```python
from build123d import *

# Parameters (mm, degrees)
ESBO_O1_R                = 2.95
RESSALTO_EXTRUS_O1_DEPTH = 1.4
CORTE_EXTRUS_O1_START    = -1
CORTE_EXTRUS_O1_DEPTH    = 1
ESBO_O3_R                = 2.1
RESSALTO_EXTRUS_O2_DEPTH = 1
FILETE3_R                = 0.2
ESBO_O4_R                = 2
RESSALTO_EXTRUS_O3_DEPTH = 6.5
FILETE4_R                = 0.2


with BuildPart() as part:
    # Esboço1 → Ressalto-extrusão1 (new body)
    with BuildSketch(Plane(origin=(0, 0, 0), x_dir=(1, 0, 0), z_dir=(0, 1, 0))):
        with Locations(Location((0, 0, 0), (0, 0, 270))):
            Circle(ESBO_O1_R)
    extrude(amount=RESSALTO_EXTRUS_O1_DEPTH)

    # Esboço2 → Corte-extrusão1 (cut)
    with BuildSketch(Plane(origin=(0, 1.4, 0), x_dir=(1, 0, 0), z_dir=(0, 1, 0)).offset(CORTE_EXTRUS_O1_START)):
        with BuildLine():
            Line((-0.25, 2.939387691), (0, 2.5))
            Line((0, 2.5), (0.25, 2.939387691))
            ThreePointArc((0.25, 2.939387691), (0, 2.95), (-0.25, 2.939387691))
        make_face()
        with BuildLine():
            Line((1.016841608, 2.283863644), (1.423943047, 2.583580113))
            ThreePointArc((1.423943047, 2.583580113), (1.199873097, 2.6949591), (0.967170318, 2.786948434))
            Line((0.967170318, 2.786948434), (1.016841608, 2.283863644))
        make_face()
        with BuildLine():
            Line((1.857862064, 1.672826516), (2.351673404, 1.781048062))
            ThreePointArc((2.351673404, 1.781048062), (2.192277235, 1.973935289), (2.017108101, 2.152620475))
            Line((2.017108101, 2.152620475), (1.857862064, 1.672826516))
        make_face()
        with BuildLine():
            Line((2.377641291, 0.772542486), (2.872778066, 0.670556621))
            ThreePointArc((2.872778066, 0.670556621), (2.805616723, 0.911600133), (2.718269569, 1.146084879))
            Line((2.718269569, 1.146084879), (2.377641291, 0.772542486))
        make_face()
        with BuildLine():
            Line((2.486304738, -0.261321158), (2.897153302, -0.555880152))
            ThreePointArc((2.897153302, -0.555880152), (2.933839591, -0.308358967), (2.949417534, -0.058619204))
            Line((2.949417534, -0.058619204), (2.486304738, -0.261321158))
        make_face()
        with BuildLine():
            Line((2.165063509, -1.25), (2.420584412, -1.686200197))
            ThreePointArc((2.420584412, -1.686200197), (2.554774941, -1.475), (2.670584412, -1.253187495))
            Line((2.670584412, -1.253187495), (2.165063509, -1.25))
        make_face()
        with BuildLine():
            Line((1.469463131, -2.022542486), (1.525474487, -2.524960908))
            ThreePointArc((1.525474487, -2.524960908), (1.733966494, -2.386600133), (1.929982984, -2.231068282))
            Line((1.929982984, -2.231068282), (1.469463131, -2.022542486))
        make_face()
        with BuildLine():
            Line((0.519779227, -2.445369002), (0.366596165, -2.927132941))
            ThreePointArc((0.366596165, -2.927132941), (0.613339488, -2.885535422), (0.855669965, -2.823177095))
            Line((0.855669965, -2.823177095), (0.519779227, -2.445369002))
        make_face()
        with BuildLine():
            Line((-0.519779227, -2.445369002), (-0.855669965, -2.823177095))
            ThreePointArc((-0.855669965, -2.823177095), (-0.613339488, -2.885535422), (-0.366596165, -2.927132941))
            Line((-0.366596165, -2.927132941), (-0.519779227, -2.445369002))
        make_face()
        with BuildLine():
            Line((-1.469463131, -2.022542486), (-1.929982984, -2.231068282))
            ThreePointArc((-1.929982984, -2.231068282), (-1.733966494, -2.386600133), (-1.525474487, -2.524960908))
            Line((-1.525474487, -2.524960908), (-1.469463131, -2.022542486))
        make_face()
        with BuildLine():
            Line((-2.165063509, -1.25), (-2.670584412, -1.253187495))
            ThreePointArc((-2.670584412, -1.253187495), (-2.554774941, -1.475), (-2.420584412, -1.686200197))
            Line((-2.420584412, -1.686200197), (-2.165063509, -1.25))
        make_face()
        with BuildLine():
            Line((-2.486304738, -0.261321158), (-2.949417534, -0.058619204))
            ThreePointArc((-2.949417534, -0.058619204), (-2.933839591, -0.308358967), (-2.897153302, -0.555880152))
            Line((-2.897153302, -0.555880152), (-2.486304738, -0.261321158))
        make_face()
        with BuildLine():
            Line((-2.377641291, 0.772542486), (-2.718269569, 1.146084879))
            ThreePointArc((-2.718269569, 1.146084879), (-2.805616723, 0.911600133), (-2.872778066, 0.670556621))
            Line((-2.872778066, 0.670556621), (-2.377641291, 0.772542486))
        make_face()
        with BuildLine():
            Line((-1.857862064, 1.672826516), (-2.017108101, 2.152620475))
            ThreePointArc((-2.017108101, 2.152620475), (-2.192277235, 1.973935289), (-2.351673404, 1.781048062))
            Line((-2.351673404, 1.781048062), (-1.857862064, 1.672826516))
        make_face()
        with BuildLine():
            Line((-1.016841608, 2.283863644), (-0.967170318, 2.786948434))
            ThreePointArc((-0.967170318, 2.786948434), (-1.199873097, 2.6949591), (-1.423943047, 2.583580113))
            Line((-1.423943047, 2.583580113), (-1.016841608, 2.283863644))
        make_face()
    extrude(amount=CORTE_EXTRUS_O1_DEPTH, mode=Mode.SUBTRACT)

    # Esboço3 → Ressalto-extrusão2 (add)
    with BuildSketch(Plane(origin=(0, 1.4, 0), x_dir=(1, 0, 0), z_dir=(0, 1, 0))):
        with Locations(Location((0, 0, 0), (0, 0, 270))):
            Circle(ESBO_O3_R)
    extrude(amount=RESSALTO_EXTRUS_O2_DEPTH)

    # Filete3
    filete3_edges = [part.edges().sort_by_distance(p)[0] for p in [
        (0, 2.4, -2.1),
    ]]
    fillet(filete3_edges, radius=FILETE3_R)

    # Esboço4 → Ressalto-extrusão3 (add)
    with BuildSketch(Plane(origin=(0, 2.4, 0), x_dir=(1, 0, 0), z_dir=(0, 1, 0))):
        with Locations(Location((0, 0, 0), (0, 0, 270))):
            Circle(ESBO_O4_R)
    extrude(amount=RESSALTO_EXTRUS_O3_DEPTH)

    # Filete4
    filete4_edges = [part.edges().sort_by_distance(p)[0] for p in [
        (0, 8.9, -2),
    ]]
    fillet(filete4_edges, radius=FILETE4_R)


solid = part.part
```
Design review of the part built by this model. Coordinates are the model's own, in mm. A direction names the side the tool comes from. Give positions to 0.01 mm unless a question says otherwise; leave off trailing zeros. Write each loop counter-clockwise with the first axis right and the second up, starting at its lowest first coordinate (ties: lowest second). Pieces come first, ordered by that corner, then holes. Notation, with made-up numbers: (16.25, 66.25) - (40.25, 66.25) arc R19 cw to (40.25, 86.25) - close; hole circle Ø1 at (48.5, 4). An arc over 180 degrees is marked (long way). Return JSON: item names as keys, results as strings. Group by question number.
(1) Machinability: for faces 1 (the flat face through (0, 0, 0)), 2 (the cylindrical face through (-2, 6, 0)), which of the approach directions +Z, -Z, +X, -X, +Y, -Y give a long, thin tool a straight path to every point of the face, cutting with its end or side? Answer none if there is none.
(2) Insertion check: pin 1 (3 mm diameter, centred on x = -1.5, y = 6.5, fed in from +Z); pin 2 (1 mm diameter, centred on x = -2, y = 2.5, fed in from -Z); pin 3 (0.5 mm diameter, centred on x = -2.5, z = 1.5, fed in from +Y). Each pin has a flat end and moves straight along its axis. Give the tip position at first contact, or say it passes through.
(3) To check wall thickness, follow probe 1 along Y at (x, z) = (2.25, 1.8); probe 2 along Y at (x, z) = (-1.95, -1.75); probe 3 along Z at (x, y) = (0.4, 5.5). State the ranges of each line that lie inside material, in increasing order.
(4) We need section A-A, the plane y = 8. Give the boundary of the cut face in (x, z).
Reported:
{
 "1": {"face 1": "+Z, -Z, +X, -X, -Y", "face 2": "+Y"},
 "2": {"pin 1": "stops at z = 2", "pin 2": "stops at z = -1.39", "pin 3": "stops at y = 1.4"},
 "3": {"probe 1": "y = 0 to 1.4", "probe 2": "y = 0 to 0.4", "probe 3": "z = -1.96 to 1.96"},
 "4": {"outline": "circle Ø4 at (0, 0)"}
}
